Part model, mm, in its own coordinate system. A direction names the side the tool comes from. Round coordinates to 2 decimals unless told otherwise and drop trailing zeros. Loops run counter-clockwise (first coordinate to the right, second up) from the corner with the lowest first, then second, coordinate; pieces in that order, holes last. Notation, with made-up numbers: (25.5, -1.5) - (59.5, -1.5) arc R30 ccw to (59.5, 32.5) - close; hole circle Ø10 at (5.5, 37). An arc over 180 degrees is marked (long way). Put each result on its own line as item: value.
from build123d import *

# Parameters (mm, degrees)
SKETCH1_R           = 12.5
SKETCH1_R_2         = 0.8
BOSS_EXTRUDE1_DEPTH = 1
BOSS_EXTRUDE2_DEPTH = 0.5


with BuildPart() as part:
    # Sketch1 → Boss-Extrude1 (new body)
    with BuildSketch(Plane(origin=(0, 0, 0), x_dir=(1, 0, 0), z_dir=(0, 1, 0))):
        with Locations(Location((0, 0, 0), (0, 0, 270))):
            Circle(SKETCH1_R)
        with Locations(Location((0, 6.25, 0), (0, 0, 270))):
            Circle(SKETCH1_R_2, mode=Mode.SUBTRACT)
        with Locations(Location((0, -6.25, 0), (0, 0, 270))):
            Circle(SKETCH1_R_2, mode=Mode.SUBTRACT)
    extrude(amount=-BOSS_EXTRUDE1_DEPTH)

    # Sketch2 → Boss-Extrude2 (add, symmetric)
    with BuildSketch(Plane.XY):
        Polygon((-11, 0), (-11, 0.721206206), (-6.5, 6.4), (-6.5, 14), (6.5, 14), (6.5, 6.4), (11, 0.721206206), (11, 0), align=None)
    extrude(amount=BOSS_EXTRUDE2_DEPTH, both=True)


solid = part.part
1. Probe line 1 along Y through (x, z) = (5, -8.5); line 2 along Z through (x, y) = (-7.5, 4.5); line 3 along X through (y, z) = (-0.5, -6.25). List the from-to ranges inside material, lowest first. Write a range as [from, to].
A:
line 1: y = [-1, 0]
line 2: z = [-0.5, 0.5]
line 3: x = [-10.83, -0.8], [0.8, 10.83]
2. Band-saw the part on A-A (x = 0). List the corners of the cut face in (y, z), plus the area to 3 significant figures.
A:
outline: (-1, -12.5) - (0, -12.5) - (0, -7.05) - (-1, -7.05) - close; (-1, -5.45) - (0, -5.45) - (0, -0.5) - (14, -0.5) - (14, 0.5) - (0, 0.5) - (0, 5.45) - (-1, 5.45) - close; (-1, 7.05) - (0, 7.05) - (0, 12.5) - (-1, 12.5) - close
area: 35.8 mm²
3. Pin check, flat tips, straight feed: P1, Ø1, axis at x = 5, y = 10, coming from the -Z side; P2, Ø0.6, axis at y = 0.5, z = 0, coming from the -X side; P3, Ø1.5, axis at y = 1, z = 7.5, coming from the -X side; P4, Ø0.8, axis at y = 0.5, z = 0, coming from the +X side. Stop position of each tip, or through.
A:
P1: stops at z = -0.5
P2: stops at x = -11
P3: passes through
P4: stops at x = 11
4. Band-saw the part on D-D (x = 2.75). List the corners of the cut face in (y, z), plus the area to 3 significant figures.
A:
outline: (-1, -12.19) - (0, -12.19) - (0, -0.5) - (14, -0.5) - (14, 0.5) - (0, 0.5) - (0, 12.19) - (-1, 12.19) - close
area: 38.4 mm²
5. Band-saw the part on B-B (z = 0). List the corners of the cut face in (x, y), plus the area to 3 significant figures.
A:
outline: (-12.5, -1) - (12.5, -1) - (12.5, 0) - (11, 0) - (11, 0.72) - (6.5, 6.4) - (6.5, 14) - (-6.5, 14) - (-6.5, 6.4) - (-11, 0.72) - (-11, 0) - (-12.5, 0) - close
area: 239 mm²
6. Tool access for faces 1 (the flat face through (0, 6, -0.5)), 2 (the flat face through (0, 6, 0.5)), 3 (the flat face through (-6.5, 10, 0)): list every direction of +Z, -Z, +X, -X, +Y, -Y with a clear straight run to the whole face (end or side of a thin tool).
A:
face 1: -Z, +X, -X, +Y
face 2: +Z, +X, -X, +Y
face 3: +Z, -Z, -X, +Y
7. Band-saw the part on C-C (z = 6.5). List the corners of the cut face in (x, y), plus the area to 3 significant figures.
A:
outline: (-10.68, -1) - (-0.76, -1) - (-0.76, 0) - (-10.68, 0) - close; (0.76, -1) - (10.68, -1) - (10.68, 0) - (0.76, 0) - close
area: 19.8 mm²
8. Two-plate mould, pull along Z, no slides. Class faces 4 (the cylindrical face through (0.04, -0.49, 5.45)), 5 (the flat face through (0, -1, 0)), 6 (the cylindrical face through (3.755, -0.493, 11.923)): pulls with the +Z half, pulls with the -Z half, needs draft (parallel to the pull), parting line crosses it, or undercut.
A:
face 4: undercut
face 5: needs draft
face 6: parting line crosses it
